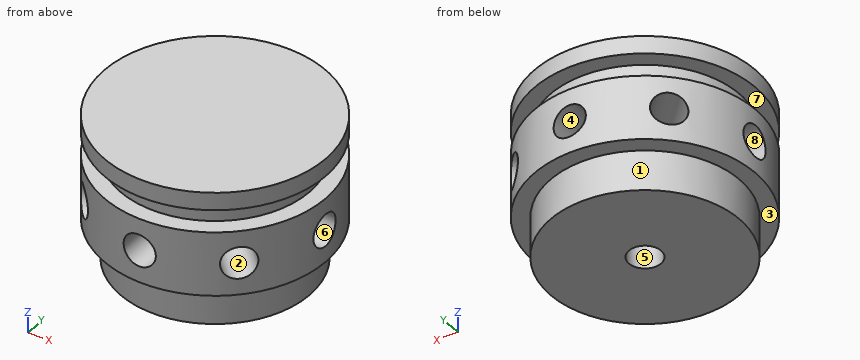
from build123d import *

# Parameters (mm, degrees)
ESBO_O3_R             = 2
CORTE_EXTRUS_O1_DEPTH = 8
PADR_OCIRCULAR1_COUNT = 8
ESBO_O4_R             = 2
CORTE_EXTRUS_O2_DEPTH = 5


with BuildPart() as part:
    # Esboço2 → Revolução1 (revolve)
    with BuildSketch(Plane(origin=(0, 0, 0), x_dir=(1, 0, 0), z_dir=(0, 1, 0)), mode=Mode.PRIVATE) as revolu_o1_sk:
        Polygon((0, 0), (-13.75, 0), (-13.75, 2.2), (-11.75, 2.2), (-11.75, 5), (-13.75, 5), (-13.75, 13), (-11.75, 13), (-11.75, 18), (0, 18), align=None)
    revolve(revolu_o1_sk.sketch.rotate(Axis((0, 0, 0), (0, 0, -1)), 180), axis=Axis((0, 0, 0), (0, 0, -1)))

    # Esboço3 → Corte-extrusão1 (cut)
    with BuildSketch(Plane(origin=(0, 13.75, 0), x_dir=(1, 0, 0), z_dir=(0, 1, 0))):
        with Locations(Location((0, 9, 0), (0, 0, 270))):
            Circle(ESBO_O3_R)
    corte_extrus_o1 = extrude(amount=-CORTE_EXTRUS_O1_DEPTH, mode=Mode.SUBTRACT)

    # PadrãoCircular1: Corte-extrusão1 ×8 about axis
    padr_ocircular1_axis = Axis((0, 0, 0), (0, 0, 1))
    for i in range(1, PADR_OCIRCULAR1_COUNT):
        add(corte_extrus_o1.rotate(padr_ocircular1_axis, i * 360 / PADR_OCIRCULAR1_COUNT), mode=Mode.SUBTRACT)

    # Esboço4 → Corte-extrusão2 (cut)
    with BuildSketch(Plane(origin=(0, 0, -18), x_dir=(-1, 0, 0), z_dir=(0, 0, -1))):
        Circle(ESBO_O4_R)
    extrude(amount=-CORTE_EXTRUS_O2_DEPTH, mode=Mode.SUBTRACT)


solid = part.part
Source: CAD feature listing. Evaluate the final solid. Frame: model axes, mm. Face numbers are marked on the shaded views. A direction names the side the tool comes from. Give positions to 0.01 mm unless a question says otherwise; leave off trailing zeros. Write each loop counter-clockwise with the first axis right and the second up, starting at its lowest first coordinate (ties: lowest second). Pieces come first, ordered by that corner, then holes. Notation, with made-up numbers: (48, 16) -> (107, 16) arc R25 ccw to (107, 43) -> close; hole circle Ø6 at (30.25, 41). An arc over 180 degrees is marked (long way). Write item = value, one per line.
Q1. Cut plane A-A on y = 0. Return loops of the section in (x, z).
Here are the results:
outline = (-13.75, -13) -> (-11.75, -13) -> (-11.75, -18) -> (-2, -18) -> (-2, -13) -> (2, -13) -> (2, -18) -> (11.75, -18) -> (11.75, -13) -> (13.75, -13) -> (13.75, -11) -> (5.75, -11) -> (5.75, -7) -> (13.75, -7) -> (13.75, -5) -> (11.75, -5) -> (11.75, -2.2) -> (13.75, -2.2) -> (13.75, 0) -> (-13.75, 0) -> (-13.75, -2.2) -> (-11.75, -2.2) -> (-11.75, -5) -> (-13.75, -5) -> (-13.75, -7) -> (-5.75, -7) -> (-5.75, -11) -> (-13.75, -11) -> close
Q2. Cut plane D-D on y = -6.5. State how many separate pieces and enclosed holes the cut face has, then the cut area to 3 significant figures.
Here are the results:
separate_pieces = 1
enclosed_holes = 3
area = 352 mm²
Q3. First-contact query: pin 1 (1.2 mm diameter, centred on x = 0, z = -8.5, fed in from -Y); pin 2 (3.5 mm diameter, centred on y = 0, z = -9, fed in from -X); pin 3 (3 mm diameter, centred on y = 0.5, z = -9.5, fed in from -X). Flat tips, straight axial feed; report the tip coordinate or a pass-through.
Here are the results:
pin_1 = -5.75
pin_2 = -5.75
pin_3 = -13.75
Q4. Line query: line 1 (Z direction, x = 0, y = 9.75); line 2 (Z direction, x = 1.25, y = 12.5); line 3 (Z direction, x = -4.5, y = 6.5). Output: solid intervals per line, ascending. Write a range as from..to.
Here are the results:
line_1 = -18..-11, -7..0
line_2 = -13..-10.56, -7.44..-5, -2.2..0
line_3 = -18..-10.41, -7.59..0
Q5. Mould query, pull axis Y, two halves, no side actions, for the marked faces 1, 2 and 3. Classes: +Y half, -Y half, draft (parallel to the pull), parting line (faces both ways), or undercut.
Here are the results:
face_1 = parting line
face_2 = undercut
face_3 = draft
Q6. Reachability of the marked faces 4, 5, 6, 7 and 8 from +Z, -Z, +X, -X, +Y, -Y: full face, straight path, thin tool, end or side. Return the list, or none.
Here are the results:
face_4 = +Y
face_5 = -Z
face_6 = +X
face_7 = none
face_8 = -X
